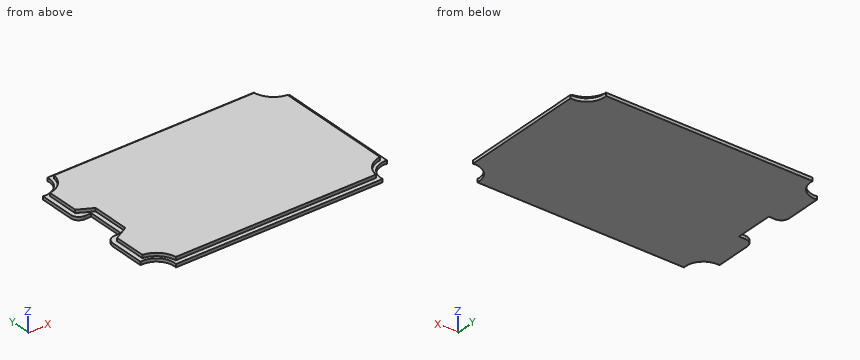
Autodesk Inventor part; units mm, degrees
ref_plane "YZ Plane" through (0, 0, 0) normal (1, 0, 0) x (0, 1, 0)
ref_plane "XZ Plane" through (0, 0, 0) normal (0, 1, 0) x (-1, 0, 0)
ref_plane "XY Plane" through (0, 0, 0) normal (0, 0, 1) x (1, 0, 0)
sketch "Sketch1" plane through (0, 0, 0) normal (0, 0, 1) x (1, 0, 0)
  line L0 (-43.5443, 19.427) -> (49.4557, 19.427)
  line L1 (52.4557, 16.427) -> (52.4557, -43.573)
  line L2 (49.4557, -46.573) -> (-43.5443, -46.573)
  line L3 (-46.5443, -43.573) -> (-46.5443, 16.427)
  arc A0 (-43.5443, 19.427) -> (-46.5443, 16.427) centre (-43.5443, 16.427) ccw
  arc A1 (-46.5443, -43.573) -> (-43.5443, -46.573) centre (-43.5443, -43.573) ccw
  arc A2 (49.4557, -46.573) -> (52.4557, -43.573) centre (49.4557, -43.573) ccw
  arc A3 (52.4557, 16.427) -> (49.4557, 19.427) centre (49.4557, 16.427) ccw
  point P0 (0, 0)
  point P1 (0, 0)
  point P2 (-46.5443, 19.427)
  point P3 (52.4557, -46.573)
  point P4 (52.4557, 19.427)
  dimension "d0" = 99
  dimension "d1" = 66
  dimension "d2" = 3
extrude "Extrusion1" add sketch "Sketch1" along normal blind 1.27
sketch "Sketch2" plane through (0, 0, 1.27) normal (0, 0, 1) x (1, 0, 0)
  line L0 (-46.5443, 16.427) -> (-46.5443, -43.573)
  line L1 (49.4557, 19.427) -> (-43.5443, 19.427)
  circle A0 centre (-42.7343, 15.617) radius 1.5875
  line L2 (-50.0562, -13.573) -> (79.0191, -13.573) construction
  line L3 (2.9557, 30.2203) -> (2.9557, -48.7988) construction
  circle A1 centre (-42.7343, -42.763) radius 1.5875
  circle A2 centre (48.6457, 15.617) radius 1.5875
  circle A3 centre (48.6457, -42.763) radius 1.5875
  point P0 (0, 0)
  dimension "d8" = 3.175
  dimension "d9" = 3.81
  dimension "d10" = 3.81
extrude "Extrusion2" cut sketch "Sketch2" against normal blind 25.4
sketch "Sketch3" plane through (0, 0, 1.27) normal (0, 0, 1) x (1, 0, 0)
  circle A0 centre (48.6457, 15.617) radius 1.5875
  circle A1 centre (-42.7343, 15.617) radius 1.5875
  circle A2 centre (-42.7343, -42.763) radius 1.5875
  circle A3 centre (48.6457, -42.763) radius 1.5875
  line L0 (49.4557, 19.427) -> (-43.5443, 19.427)
  arc A4 (-43.5443, 19.427) -> (-46.5443, 16.427) centre (-43.5443, 16.427) ccw
  line L1 (-46.5443, 16.427) -> (-46.5443, -43.573) construction
  arc A5 (-46.5443, -43.573) -> (-43.5443, -46.573) centre (-43.5443, -43.573) ccw
  line L2 (-43.5443, -46.573) -> (49.4557, -46.573)
  arc A6 (49.4557, -46.573) -> (52.4557, -43.573) centre (49.4557, -43.573) ccw
  line L3 (52.4557, -43.573) -> (52.4557, 16.427)
  arc A7 (52.4557, 16.427) -> (49.4557, 19.427) centre (49.4557, 16.427) ccw
  arc A8 (-43.5443, 19.427) -> (-46.5443, 16.427) centre (-43.5443, 16.427) ccw
  line L4 (49.4557, 19.427) -> (-43.5443, 19.427)
  circle A9 centre (48.6457, 15.617) radius 1.5875
  circle A10 centre (-42.7343, 15.617) radius 1.5875
  circle A11 centre (-42.7343, -42.763) radius 1.5875
  circle A12 centre (48.6457, -42.763) radius 1.5875
  arc A13 (52.4557, 16.427) -> (49.4557, 19.427) centre (49.4557, 16.427) ccw
  line L5 (52.4557, 16.427) -> (52.4557, -43.573)
  arc A14 (49.4557, -46.573) -> (52.4557, -43.573) centre (49.4557, -43.573) ccw
  line L6 (49.4557, -46.573) -> (-43.5443, -46.573)
  arc A15 (-46.5443, -43.573) -> (-43.5443, -46.573) centre (-43.5443, -43.573) ccw
  line L7 (-46.5443, -43.573) -> (-46.5443, 16.427)
  arc A16 (-43.5443, 19.427) -> (-46.5443, 16.427) centre (-43.5443, 16.427) ccw
  line L8 (-43.5443, 19.427) -> (49.4557, 19.427)
  line L9 (-43.5443, 19.427) -> (49.4557, 19.427)
  line L10 (-40.8039, 19.427) -> (-40.8039, -46.573) construction
  line L11 (49.4557, -46.573) -> (-43.5443, -46.573)
  line L12 (-40.8039, 19.427) -> (-51.3078, 19.427) construction
  line L13 (-40.8039, -46.573) -> (-51.3078, -46.573) construction
  line L14 (-40.8039, -21.173) -> (-51.3078, -21.173) construction
  line L15 (-40.8039, -5.973) -> (-51.3078, -5.973) construction
  line L16 (-46.5443, -43.573) -> (-46.5443, 16.427)
  line L17 (-46.5443, -5.973) -> (-40.8039, -5.973)
  line L18 (-40.8039, -5.973) -> (-40.8039, -21.173)
  line L19 (-40.8039, -21.173) -> (-46.5443, -21.173)
  line L20 (-46.5443, -21.173) -> (-46.5443, -5.973)
  point P0 (0, 0)
  dimension "d13" = 25.4
  dimension "d14" = 25.4
  dimension "d15" = 5.7404
extrude "Extrusion3" cut sketch "Sketch3" against normal blind 25.4 contours L17 L18 L19 L7
fillet "Fillet1" radius 3.175 2 edges at (-46.5443, -21.173, 0.635) (-46.5443, -5.973, 0.635)
sketch "Sketch9" plane through (0, 0, 1.27) normal (0, 0, 1) x (1, 0, 0)
  arc A0 (-43.5443, 19.427) -> (-46.5443, 16.427) centre (-43.5443, 16.427) ccw
  line L0 (-46.5443, -2.798) -> (-46.5443, 16.427) construction
  line L1 (-46.5443, 16.427) -> (-46.5443, -2.798)
  line L2 (-43.5443, 19.427) -> (-26.5771, 19.427) construction
  line L3 (49.4557, 19.427) -> (-43.5443, 19.427)
  line L4 (-45.6657, 18.5483) -> (-26.5771, -0.5403) construction
  line L5 (-45.6657, 18.5483) -> (-18.6704, 18.5483) construction
  circle A1 centre (-45.6657, 18.5483) radius 7.1603
  arc A2 (-46.5443, -2.798) -> (-43.3693, -5.973) centre (-43.3693, -2.798) ccw
  line L6 (-43.3693, -5.973) -> (-40.8039, -5.973)
  line L7 (-40.8039, -5.973) -> (-40.8039, -21.173)
  line L8 (-40.8039, -21.173) -> (-43.3693, -21.173)
  arc A3 (-43.3693, -21.173) -> (-46.5443, -24.348) centre (-43.3693, -24.348) ccw
  line L9 (-46.5443, -24.348) -> (-46.5443, -43.573)
  arc A4 (-46.5443, -43.573) -> (-43.5443, -46.573) centre (-43.5443, -43.573) ccw
  line L10 (-43.5443, -46.573) -> (49.4557, -46.573)
  arc A5 (49.4557, -46.573) -> (52.4557, -43.573) centre (49.4557, -43.573) ccw
  line L11 (52.4557, -43.573) -> (52.4557, 16.427)
  arc A6 (52.4557, 16.427) -> (49.4557, 19.427) centre (49.4557, 16.427) ccw
  line L12 (49.4557, 19.427) -> (-43.5443, 19.427)
  arc A7 (-43.5443, 19.427) -> (-46.5443, 16.427) centre (-43.5443, 16.427) ccw
  line L13 (-46.5443, 16.427) -> (-46.5443, -2.798)
  circle A8 centre (48.6457, 15.617) radius 1.5875
  circle A9 centre (-42.7343, 15.617) radius 1.5875
  circle A10 centre (-42.7343, -42.763) radius 1.5875
  circle A11 centre (48.6457, -42.763) radius 1.5875
  line L14 (-75.7777, -13.573) -> (114.1059, -13.573) construction
  line L15 (2.9557, 31.1348) -> (2.9557, -53.319) construction
  circle A12 centre (-45.6657, -45.6944) radius 7.1603
  line L16 (2.9557, -58.2809) -> (2.9557, 26.1729) construction
  circle A13 centre (51.577, 18.5483) radius 7.1603
  circle A14 centre (51.577, -45.6944) radius 7.1603
  point P0 (0, 0)
  dimension "d28" = 45
extrude "Extrusion5" cut sketch "Sketch9" against normal blind 12.7 contours L3 A1 L1 A0 | A0 L1 A1 L3 | A13 L11 A6 L3 | L3 A6 L11 A13 | A14 L10 A5 L11 | L11 A5 L10 A14 | A12 L9 A4 L10 | L10 A4 L9 A12
sketch "Sketch10" plane through (0, 0, 1.27) normal (0, 0, 1) x (1, 0, 0)
  arc A0 (52.4557, -38.5882) -> (44.4708, -46.573) centre (51.577, -45.6944) ccw
  line L0 (52.4557, -38.5882) -> (52.4557, 11.4421)
  arc A1 (44.4708, 19.427) -> (52.4557, 11.4421) centre (51.577, 18.5483) ccw
  line L1 (44.4708, 19.427) -> (-38.5595, 19.427)
  arc A2 (-46.5443, 11.4421) -> (-38.5595, 19.427) centre (-45.6657, 18.5483) ccw
  line L2 (-46.5443, 11.4421) -> (-46.5443, -2.798)
  arc A3 (-46.5443, -2.798) -> (-43.3693, -5.973) centre (-43.3693, -2.798) ccw
  line L3 (-43.3693, -5.973) -> (-40.8039, -5.973)
  line L4 (-40.8039, -5.973) -> (-40.8039, -21.173)
  line L5 (-40.8039, -21.173) -> (-43.3693, -21.173)
  arc A4 (-43.3693, -21.173) -> (-46.5443, -24.348) centre (-43.3693, -24.348) ccw
  line L6 (-46.5443, -24.348) -> (-46.5443, -38.5882)
  arc A5 (-38.5595, -46.573) -> (-46.5443, -38.5882) centre (-45.6657, -45.6944) ccw
  line L7 (-38.5595, -46.573) -> (44.4708, -46.573)
  line L8 (-36.7645, -44.795) -> (43.1467, -44.795)
  line L9 (-36.7645, 17.649) -> (43.1467, 17.649)
  line L10 (44.4708, 19.427) -> (-38.5595, 19.427)
  line L11 (-36.7645, -44.795) -> (-37.2354, -44.795)
  arc A6 (-38.5595, -46.573) -> (-46.5443, -38.5882) centre (-45.6657, -45.6944) ccw
  line L12 (-36.7645, 17.649) -> (-37.2354, 17.649)
  line L13 (50.6777, 10.118) -> (50.6777, -37.264)
  arc A7 (44.4708, 19.427) -> (52.4557, 11.4421) centre (51.577, 18.5483) ccw
  line L14 (-39.0259, -5.973) -> (-39.0259, -21.173)
  line L15 (-44.7663, -2.798) -> (-39.0259, -5.973)
  line L16 (-39.0259, -21.173) -> (-44.7663, -24.348)
  line L17 (50.6777, 10.118) -> (52.4557, 10.118) construction
  line L18 (52.4557, -38.5882) -> (52.4557, 11.4421)
  line L19 (43.1467, 17.649) -> (43.1467, 19.427) construction
  arc A8 (43.1467, 17.649) -> (50.6777, 10.118) centre (51.7594, 18.7307) ccw
  line L20 (-56.5649, -13.573) -> (80.9191, -13.573) construction
  line L21 (2.9557, 34.2968) -> (2.9557, -68.6615) construction
  arc A9 (50.6777, -37.264) -> (43.1467, -44.795) centre (51.7594, -45.8768) ccw
  arc A10 (-44.7663, 10.118) -> (-37.2354, 17.649) centre (-45.8481, 18.7307) ccw
  arc A11 (-37.2354, -44.795) -> (-44.7663, -37.264) centre (-45.8481, -45.8768) ccw
  line L22 (-44.7663, 10.118) -> (-44.7663, -2.798)
  line L23 (-44.7663, -37.264) -> (-44.7663, -24.348)
  line L24 (-46.5443, -43.573) -> (-46.5443, -24.348)
  point P0 (0, 0)
  dimension "d31" = 1.778
  dimension "d32" = 1.778
  dimension "d35" = 1.778
  dimension "d36" = 1.778
  dimension "d39" = 3.175
  dimension "d40" = 3.175
  dimension "d42" = 1.27
  dimension "d43" = 1.27
  dimension "d44" = 1.778
  dimension "d56" = 1.778
extrude "Extrusion6" cut sketch "Sketch10" against normal blind 7.62 contours L11 A11 L23 L16 L14 L15 L22 A10 L12 L9 A8 L13 A9 L8
sketch "Sketch13" plane through (0, 0, 1.27) normal (0, 0, 1) x (1, 0, 0)
  arc A0 (50.6777, -37.264) -> (43.1467, -44.795) centre (51.7594, -45.8768) ccw
  line L0 (43.1467, -44.795) -> (-37.2354, -44.795)
  arc A1 (-37.2354, -44.795) -> (-44.7663, -37.264) centre (-45.8481, -45.8768) ccw
  line L1 (-44.7663, -37.264) -> (-44.7663, -24.348)
  line L2 (-44.7663, -24.348) -> (-39.0259, -21.173)
  line L3 (-39.0259, -21.173) -> (-39.0259, -5.973)
  line L4 (-39.0259, -5.973) -> (-44.7663, -2.798)
  line L5 (-44.7663, -2.798) -> (-44.7663, 10.118)
  arc A2 (-44.7663, 10.118) -> (-37.2354, 17.649) centre (-45.8481, 18.7307) ccw
  line L6 (-37.2354, 17.649) -> (43.1467, 17.649)
  arc A3 (43.1467, 17.649) -> (50.6777, 10.118) centre (51.7594, 18.7307) ccw
  line L7 (50.6777, 10.118) -> (50.6777, -37.264)
  arc A4 (52.4557, -38.5882) -> (44.4708, -46.573) centre (51.577, -45.6944) ccw
  line L8 (52.4557, -38.5882) -> (52.4557, 11.4421)
  arc A5 (44.4708, 19.427) -> (52.4557, 11.4421) centre (51.577, 18.5483) ccw
  line L9 (44.4708, 19.427) -> (-38.5595, 19.427)
  arc A6 (-46.5443, 11.4421) -> (-38.5595, 19.427) centre (-45.6657, 18.5483) ccw
  line L10 (-46.5443, 11.4421) -> (-46.5443, -2.798)
  arc A7 (-46.5443, -2.798) -> (-43.3693, -5.973) centre (-43.3693, -2.798) ccw
  line L11 (-43.3693, -5.973) -> (-40.8039, -5.973)
  line L12 (-40.8039, -5.973) -> (-40.8039, -21.173)
  line L13 (-40.8039, -21.173) -> (-43.3693, -21.173)
  arc A8 (-43.3693, -21.173) -> (-46.5443, -24.348) centre (-43.3693, -24.348) ccw
  line L14 (-46.5443, -24.348) -> (-46.5443, -38.5882)
  arc A9 (-38.5595, -46.573) -> (-46.5443, -38.5882) centre (-45.6657, -45.6944) ccw
  line L15 (-38.5595, -46.573) -> (44.4708, -46.573)
  point P0 (0, 0)
extrude "Extrusion9" add sketch "Sketch13" along normal blind 1.27 and the other way blind 1.27 contours A0 L0 A1 L1 L2 L3 L4 L5 A2 L6 A3 L7
properties part number "battbase_lid-shrink_final"
CAD build for the part. Positions are in the model's coordinates, mm. Round coordinates to 2 decimals unless told otherwise and drop trailing zeros. Write each loop counter-clockwise with the first axis right and the second up, starting at its lowest first coordinate (ties: lowest second). Pieces come first, ordered by that corner, then holes. Notation, with made-up numbers: (33.25, -2.75) -> (53.25, -2.75) arc R17 cw to (53.25, 1.25) -> close; hole circle Ø7 at (30, 13.25). An arc over 180 degrees is marked (long way). Answer as a JSON object with one key per item and string values.
(1) Probe probe 1 along X at (y, z) = (-6.5, 0.4); probe 2 along X at (y, z) = (-36, 2.2); probe 3 along Y at (x, z) = (42, 1.6) (3 decimals). List the from-to ranges inside material, lowest first. Write a range as [from, to].
Reported:
{"probe 1": "x = [-40.8, 52.46]", "probe 2": "x = [-44.77, 50.68]", "probe 3": "y = [-44.795, 17.649]"}
(2) Band-saw the part on A-A, the plane x = 19.5. List the corners of the cut face in (y, z) (3 decimals).
Reported:
{"outline": "(-46.573, 0) -> (19.427, 0) -> (19.427, 1.27) -> (17.649, 1.27) -> (17.649, 2.54) -> (-44.795, 2.54) -> (-44.795, 1.27) -> (-46.573, 1.27) -> close"}
(3) Band-saw the part on C-C, the plane z = 2.1. List the corners of the cut face in (x, y) (1 decimal).
Reported:
{"outline": "(-44.8, -37.3) arc R8.7 cw to (-37.2, -44.8) -> (43.1, -44.8) arc R8.7 cw to (50.7, -37.3) -> (50.7, 10.1) arc R8.7 cw to (43.1, 17.6) -> (-37.2, 17.6) arc R8.7 cw to (-44.8, 10.1) -> (-44.8, -2.8) -> (-39, -6) -> (-39, -21.2) -> (-44.8, -24.3) -> close"}
(4) Band-saw the part on B-B, the plane y = 5. List the corners of the cut face in (x, z), then the cut area to 3 significant figures.
Reported:
{"outline": "(-46.54, 0) -> (52.46, 0) -> (52.46, 1.27) -> (50.68, 1.27) -> (50.68, 2.54) -> (-44.77, 2.54) -> (-44.77, 1.27) -> (-46.54, 1.27) -> close", "area": "247 mm^2"}
(5) Pin check, flat tips, straight feed: P1, Ø1.4, axis at y = -28, z = 2, coming from the -X side; P2, Ø1.4, axis at y = -15, z = 0.5, coming from the -X side; P3, Ø0.6, axis at x = -42, z = 0.5, coming from the -Y side. Stop position of each tip, or through.
Reported:
{"P1": "stops at x = -44.77", "P2": "stops at x = -40.8", "P3": "stops at y = -39.73"}
